The figure shows three views and two pictorial views of one solid part (mm, origin at its lowest corner). Answer the questions. A direction names the side the tool comes from. Give positions to 0.01 mm unless a question says otherwise; leave off trailing zeros. Loops run counter-clockwise (first coordinate to the right, second up) from the corner with the lowest first, then second, coordinate; pieces in that order, holes last. Notation, with made-up numbers: M 35,18.25 L 89,18.25 A13 ccw 89,35.25 Z; hole C -2,51 d8. An arc over 180 degrees is marked long. Write item = value, one per line. Start each with the question number.
1. Section A-A on x = 4 is taken. Determine the outline of the cut face in (y, z) (3 decimals), plus the area to 3 significant figures.
2. Consider L1, parallel to X at y = 8.5, z = 1; L2, parallel to Z at x = 4.75, y = 8.5; L3, parallel to Y at x = 4.75, z = 0.75. Determine where each line is inside the solid, lowest interval first. Write a range as [from, to].
3. Section B-B on z = 7 is taken. Determine the outline of the cut face in (x, y).
4. Flat-ended cylindrical pins translate along their axes: pin 1 Ø4 at (x, y) = (1, 21.5) entering from +Z; pin 2 Ø0.8 at (y, z) = (5.5, 1) entering from -X; pin 3 Ø3 at (x, y) = (7, 19) entering from -Z; pin 4 Ø2 at (x, z) = (4, 1.5) entering from -Y. Find the tip coordinate at first contact, or state that the pin passes through.
5. Section D-D on y = 12.75 is taken. Determine the outline of the cut face in (x, z) (3 decimals).
6. Section C-C on y = 9.5 is taken. Determine the outline of the cut face in (x, z), plus the area to 3 significant figures.
7. For the marked faces 1 and 2, determine the directions among +Z, -Z, +X, -X, +Y, -Y from which every point of the face is accessible in a straight line to the end or side of a thin tool.
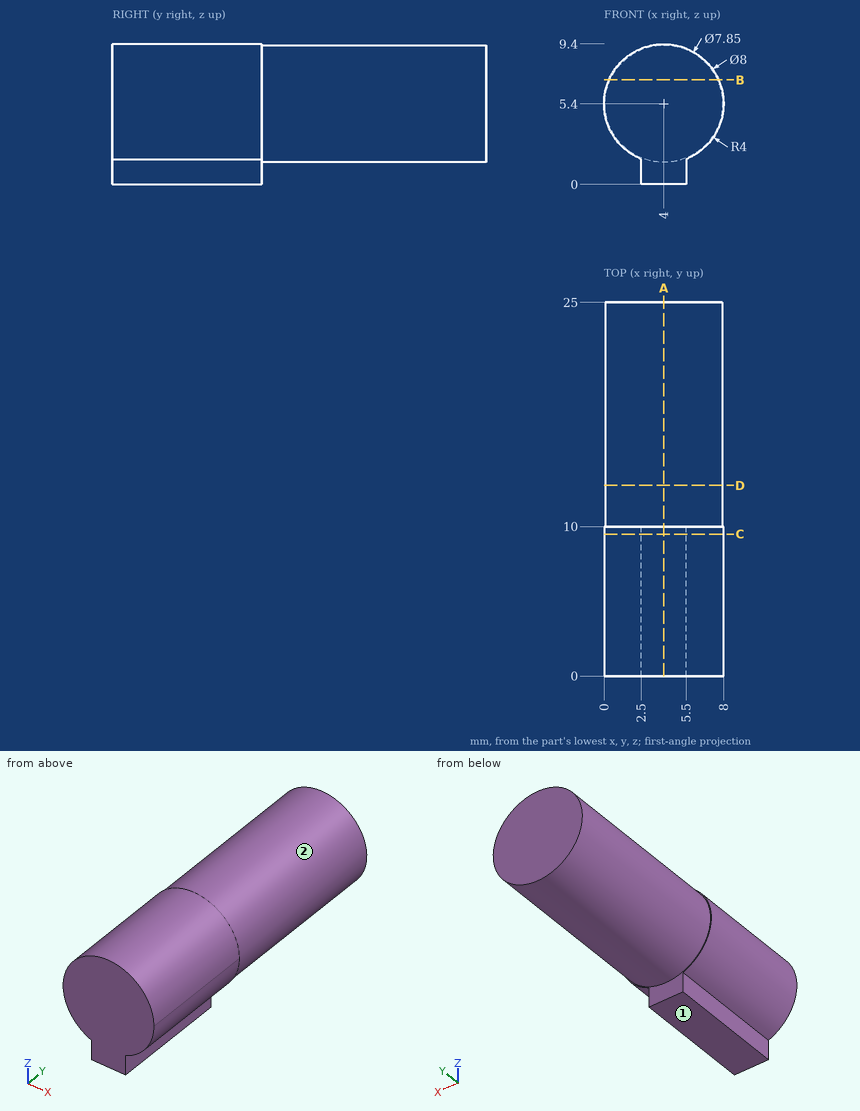
Verdict:
q1.outline = M 0,0 L 10,0 L 10,1.475 L 25,1.475 L 25,9.325 L 10,9.325 L 10,9.4 L 0,9.4 Z
q1.area = 212 mm2
q2.L1 = [2.5, 5.5]
q2.L2 = [0, 9.33]
q2.L3 = [0, 10]
q3.outline = M 0.33,0 L 7.67,0 L 7.67,10 L 7.58,10 L 7.58,25 L 0.42,25 L 0.42,10 L 0.33,10 Z
q4.pin_1 = 9.2
q4.pin_2 = 2.5
q4.pin_3 = 1.77
q4.pin_4 = 0
q5.outline = C 4,5.4 d7.85
q6.outline = M 2.5,0 L 5.5,0 L 5.5,1.69 A4 ccw long 2.5,1.69 Z
q6.area = 54.8 mm2
q7.face_1 = -Z, +X, -X, +Y, -Y
q7.face_2 = +Y
